Input: part model. Units: mm. Frame: model coordinates. Coordinates: 2 decimals unless noted, no trailing zeros. Loops run counter-clockwise (first coordinate to the right, second up) from the corner with the lowest first, then second, coordinate; pieces in that order, holes last.
(1) Contact query for flat-ended pins moving along their axis: P1, Ø6, axis at x = -72.5, y = -3.5, coming from the -Z side; P2, Ø2, axis at x = -35, z = 43, coming from the +Y side; P3, Ø12, axis at x = 79.5, y = -25, coming from the +Z side; P4, Ø8, axis at x = 1.5, y = -21.5, coming from the +Z side. Output: stop coordinate, or through.
(2) Line query: L1, parallel to Y at x = 68, z = -16; L2, parallel to Z at x = 6, y = -21.25; L3, parallel to Z at x = 0, y = -16.25. Output: solid intervals per line, ascending.
(3) Mould query, pull axis Z, two halves, no side actions, for faces 1 (the face through (-1, 0, -18)), 2 (the face through (-2.17, -12.68, -9.76)). Classes: released by +Z, released by -Z, zero draft, split by the parting line, or undercut.
(4) Section C-C, the plane y = -11.5. Return loops of the section in (x, z), then the cut area to 3 significant figures.
```python
from build123d import *

# Parameters (mm, degrees)
F0_R     = 100
F1_DEPTH = 30
F2_R     = 14.99999
F3_DEPTH = 5
F4_R     = 10
F5_DEPTH = 25.001


# Not quite as in the source:
# - a fillet or chamfer is up to 0.001 mm smaller than in the source, because OpenCascade refuses the exact size


with BuildPart() as f1:
    # F0 (on Front) → F1 (new body)
    with BuildSketch(Plane.XZ):
        Circle(F0_R)
    extrude(amount=F1_DEPTH)

    # F2 (radius 15 in the source; OpenCascade refuses exactly that, so slightly less here)
    f2_edges = [f1.edges().sort_by_distance(p)[0] for p in [
        (-100, -30, 0),
        (-100, 0, 0),
    ]]
    fillet(f2_edges, radius=F2_R)

    # F3 (cut): a face of the model
    f3_faces = [f1.faces().sort_by_distance(p)[0] for p in [
        (0, -30, 0),
    ]]
    extrude(f3_faces, amount=-F3_DEPTH, mode=Mode.SUBTRACT)

    # F4 (on face) → F5 (cut, through all)
    with BuildSketch(Plane.XZ.offset(25)):
        Circle(F4_R)
    extrude(amount=-F5_DEPTH, mode=Mode.SUBTRACT)


solid = f1.part
```
Report:
1. P1: stops at z = -66.33
1. P2: stops at y = 0
1. P3: stops at z = 64.33
1. P4: stops at z = 99.78
2. L1: y = -25 to 0
2. L2: z = -98.45 to -8, 8 to 98.45
2. L3: z = -99.95 to -10, 10 to 99.95
3. face 1: zero draft
3. face 2: undercut
4. outline: circle Ø199.17 at (0, 0); hole circle Ø20 at (0, 0)
4. area: 30,800 mm2
